The model under review builds one solid part; all positions refer to its coordinate system, in mm. Round coordinates to 2 decimals unless told otherwise and drop trailing zeros. Write each loop counter-clockwise with the first axis right and the second up, starting at its lowest first coordinate (ties: lowest second). Pieces come first, ordered by that corner, then holes. Notation, with made-up numbers: (-17, 56.5) -> (-4, 56.5) arc R23 ccw to (-4, 86.5) -> close; hole circle Ø5 at (32.25, 43). An arc over 180 degrees is marked (long way). Use CSV: the item, a comma, the result in double quotes. Start each with the question number.
1) For pin 1 Ø6 at (x, y) = (-3.5, 5) entering from -Z, flat-tipped, find the tip position at first contact; note if it passes through.
2) Wall thickness on probe 1 along X at (y, z) = (11.5, 9.75); probe 2 along Z at (x, y) = (4.5, 4); probe 3 along Z at (x, y) = (-5, 4): over which ranges is each line inside the solid? List them lowest first. Write a range as [from, to].
3) Take a section at B-B, the plane x = 2.5. Give the boundary of the cut face in (y, z).
4) Take a section at A-A, the plane y = 10. Give the boundary of the cut face in (x, z).
5) Take a section at C-C, the plane z = 5.75. Give the boundary of the cut face in (x, y).
from build123d import *

# Parameters (mm, degrees)
BOSS_EXTRUDE1_DEPTH = 15


with BuildPart() as part:
    # Sketch1 → Boss-Extrude1 (new body)
    with BuildSketch(Plane(origin=(0, 0, 0), x_dir=(1, 0, 0), z_dir=(0, 1, 0))):
        with BuildLine():
            ThreePointArc((10, -10), (7.071067812, -2.928932188), (0, 0))
            Line((0, 0), (0, -20))
            Line((0, -20), (10, -20))
            Line((10, -20), (10, -10))
        make_face()
        with BuildLine():
            Line((0, -20), (0, 0))
            ThreePointArc((0, 0), (-7.071067812, -2.928932188), (-10, -10))
            Line((-10, -10), (-10, -20))
            Line((-10, -20), (0, -20))
        make_face()
    extrude(amount=BOSS_EXTRUDE1_DEPTH)


solid = part.part
Values found:
1,pin 1,"z = 0.01"
2,probe 1,"[-10, 10]"
2,probe 2,"[1.07, 20]"
2,probe 3,"[1.34, 20]"
3,outline,"(0, 0.32) -> (15, 0.32) -> (15, 20) -> (0, 20) -> close"
4,outline,"(-10, 10) arc R10 ccw to (10, 10) -> (10, 20) -> (-10, 20) -> close"
5,outline,"(-9.05, 0) -> (9.05, 0) -> (9.05, 15) -> (-9.05, 15) -> close"
